The listing builds one solid part. Answer for the finished solid, in the listing's coordinates (mm). Face numbers are marked on the shaded views. Round coordinates to 2 decimals unless told otherwise and drop trailing zeros. Write each loop counter-clockwise with the first axis right and the second up, starting at its lowest first coordinate (ties: lowest second). Pieces come first, ordered by that corner, then holes.
from build123d import *

# Parameters (mm, degrees)
IZIM6_R                     = 15.5
IZIM6_R_2                   = 5
Y_KSEKLIK_EKSTR_ZYON2_DEPTH = 2


with BuildPart() as part:
    # Çizim5 → Döndür1 (revolve)
    with BuildSketch(Plane(origin=(0, 0, 0), x_dir=(0, 0, -1), z_dir=(1, 0, 0))):
        Polygon((12.5, 20), (15.5, 20), (29, 0), (29, -20), (26, -20), (26, 0), align=None)
    revolve(axis=Axis((0, 40.284256648, 0), (0, -1, 0)))

    # Çizim6 → Yükseklik-Ekstrüzyon2 (add)
    with BuildSketch(Plane(origin=(0, 20, 0), x_dir=(1, 0, 0), z_dir=(0, 1, 0))):
        Circle(IZIM6_R)
        with Locations((0, -7.5)):
            Circle(IZIM6_R_2, mode=Mode.SUBTRACT)
    extrude(amount=Y_KSEKLIK_EKSTR_ZYON2_DEPTH)


solid = part.part
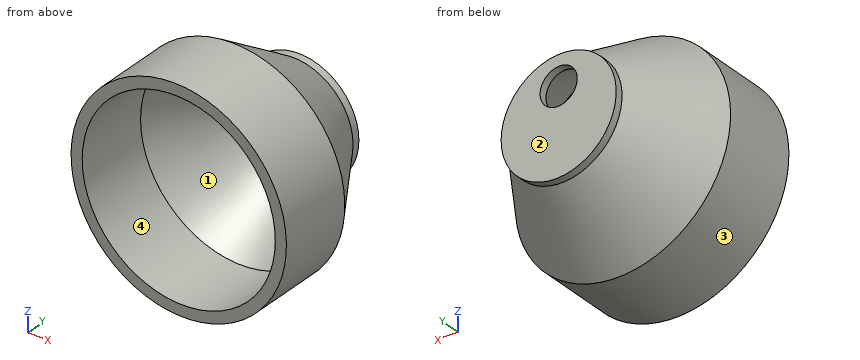
1. Given pin 1 (10 mm diameter, centred on x = -14, y = 16, fed in from -Z); pin 2 (6 mm diameter, centred on x = 11, y = 5.5, fed in from -Z); pin 3 (1.5 mm diameter, centred on x = 12, z = 21.5, fed in from +Y), each flat-ended and moving along its own axis, determine where each tip first touches the part or whether it passes through.
Geometry says:
pin 1: stops at z = -17.77
pin 2: stops at z = -25.32
pin 3: stops at y = 7.6
2. Straight lines are drawn through the part: line 1 along X through (y, z) = (-7.75, 0); line 2 along Y through (x, z) = (-2, -6); line 3 along Z through (x, y) = (-23.5, -6). For each, find the intervals that lie inside material, in ascending order.
Geometry says:
line 1: x = -29 to -26, 26 to 29
line 2: y = 20 to 22
line 3: z = -16.99 to -11.12, 11.12 to 16.99
3. Section C-C on y = 3.5 is taken. Determine the outline of the cut face in (x, z) (1 decimal).
Geometry says:
outline: circle Ø53.3 at (0, 0); hole circle Ø47.3 at (0, 0)
4. Section A-A on z = 0 is taken. Determine the outline of the cut face in (x, y), plus the area to 3 significant figures.
Geometry says:
outline: (-29, -20) - (-26, -20) - (-26, 0) - (-12.5, 20) - (12.5, 20) - (26, 0) - (26, -20) - (29, -20) - (29, 0) - (15.5, 20) - (15.5, 22) - (-15.5, 22) - (-15.5, 20) - (-29, 0) - close
area: 302 mm2
5. For a pull along Z with two mould halves and no side action, classify the marked faces 1, 2, 3 and 4 as released by +Z, released by -Z, zero draft, split by the parting line, or undercut.
Geometry says:
face 1: undercut
face 2: zero draft
face 3: split by the parting line
face 4: undercut
6. Section B-B on y = -3 is taken. Determine the outline of the cut face in (x, z).
Geometry says:
outline: circle Ø58 at (0, 0); hole circle Ø52 at (0, 0)
